from build123d import *

# Parameters (mm, degrees)
F0_W     = 584.2
F0_H     = 136.525
F1_DEPTH = 88.9
F2_R     = 3.81
F3_T     = -2.54


# Not quite as in the source:
# - a shell that OpenCascade refuses in one call is made with other operations: the cavity is built on its own and cut out


with BuildPart() as f1:
    # F0 (on Front) → F1 (new body)
    with BuildSketch(Plane.XZ):
        Rectangle(F0_W, F0_H)
    extrude(amount=F1_DEPTH)

    # F2
    f2_edges = [f1.edges().sort_by_distance(p)[0] for p in [
        (-292.1, -44.45, 68.2625),
        (0, 0, 68.2625),
        (0, -88.9, 68.2625),
        (-292.1, -88.9, 0),
        (0, -88.9, -68.2625),
        (292.1, -88.9, 0),
        (292.1, -44.45, 68.2625),
        (-292.1, 0, 0),
        (-292.1, -44.45, -68.2625),
        (0, 0, -68.2625),
        (292.1, 0, 0),
        (292.1, -44.45, -68.2625),
    ]]
    fillet(f2_edges, radius=F2_R)

    # F3: a shell. OpenCascade refuses it in one call, so the cavity is built on its own and cut out:
    # the body offset inwards by the wall thickness, plus a prism from it out through each open face.
    f3_core = offset(f1.part, amount=F3_T, mode=Mode.PRIVATE)
    f3_exits = [f3_core.faces().sort_by_distance(p)[0] for p in [
        (0, -44.45, 65.7225),
    ]]
    add(f3_core, mode=Mode.SUBTRACT)
    extrude(f3_exits, amount=-F3_T, mode=Mode.SUBTRACT)


solid = f1.part
Read the model definition and answer for the solid it produces. Units are mm, in the model's axes. A direction names the side the tool comes from. Coordinates: 2 decimals unless noted, no trailing zeros. Order: outer loops, then holes, each group sorted by start corner. A loop starts at its lowest first (then second) coordinate and runs counter-clockwise, first axis right, second up. Notation, with made-up numbers: M -39,12.25 L 11,12.25 A20 ccw 11,49.25 Z; hole C 70,-3 d5. An arc over 180 degrees is marked long. Put each result on its own line as item: value. Start each with the question number.
Item 1: Consider probe 1 along Y at (x, z) = (-238, -5.5); probe 2 along X at (y, z) = (-60, 47.5); probe 3 along Z at (x, y) = (226, -82). Determine where each line is inside the solid, lowest interval first. Write a range as [from, to].
Item 2: For faces 4 (the face through (-4, -44, -65.722)), 5 (the face through (-289.56, -44, -1)), 6 (the face through (-4, -44, -68.262)), determine the directions among +Z, -Z, +X, -X, +Y, -Y from which every point of the face is accessible in a straight line to the end or side of a thin tool.
Item 3: Section A-A, the plane z = 39.5 is taken. Determine the outline of the cut face in (x, y).
Item 4: Section C-C, the plane y = -40 is taken. Determine the outline of the cut face in (x, z), plus the area to 3 significant figures.
Item 5: The mould has two halves that part along Y. Classify faces 1 (the face through (-4, -2.54, 1)), 2 (the face through (292.1, -44, -1)), 3 (the face through (-4, -88.9, 1)): +Y half, -Y half, draft (parallel to the pull), parting line (faces both ways), or undercut.
Item 6: Section B-B, the plane x = -232.5 is taken. Determine the outline of the cut face in (y, z), plus the area to 3 significant figures.
Item 7: Given pin 1 Ø6 at (x, y) = (231, -58.5) entering from +Z; pin 2 Ø0.8 at (y, z) = (-35.5, 67.5) entering from -X; pin 3 Ø0.8 at (x, z) = (-63, 67.5) entering from -Y, each flat-ended and moving along its own axis, determine where each tip first touches the part or whether it passes through.
Computed:
1. probe 1: y = [-88.9, -86.36], [-2.54, 0]
1. probe 2: x = [-292.1, -289.56], [289.56, 292.1]
1. probe 3: z = [-68.26, -65.72]
2. face 4: +Z
2. face 5: none
2. face 6: -Z, +X, -X, +Y, -Y
3. outline: M -292.1,-85.09 A3.81 ccw -288.29,-88.9 L 288.29,-88.9 A3.81 ccw 292.1,-85.09 L 292.1,-3.81 A3.81 ccw 288.29,0 L -288.29,0 A3.81 ccw -292.1,-3.81 Z; hole M -289.56,-85.09 A1.27 ccw -288.29,-86.36 L 288.29,-86.36 A1.27 ccw 289.56,-85.09 L 289.56,-3.81 A1.27 ccw 288.29,-2.54 L -288.29,-2.54 A1.27 ccw -289.56,-3.81 Z
4. outline: M -292.1,-64.45 A3.81 ccw -288.29,-68.26 L 288.29,-68.26 A3.81 ccw 292.1,-64.45 L 292.1,64.45 A3.81 ccw 288.29,68.26 L 288.29,65.72 A1.27 cw 289.56,64.45 L 289.56,-64.45 A1.27 cw 288.29,-65.72 L -288.29,-65.72 A1.27 cw -289.56,-64.45 L -289.56,64.45 A1.27 cw -288.29,65.72 L -288.29,68.26 A3.81 ccw -292.1,64.45 Z
4. area: 2,160 mm2
5. face 1: undercut
5. face 2: draft
5. face 3: -Y half
6. outline: M -88.9,-64.45 A3.81 ccw -85.09,-68.26 L -3.81,-68.26 A3.81 ccw 0,-64.45 L 0,64.45 A3.81 ccw -3.81,68.26 L -3.81,65.72 A1.27 cw -2.54,64.45 L -2.54,-64.45 A1.27 cw -3.81,-65.72 L -85.09,-65.72 A1.27 cw -86.36,-64.45 L -86.36,64.45 A1.27 cw -85.09,65.72 L -85.09,68.26 A3.81 ccw -88.9,64.45 Z
6. area: 902 mm2
7. pin 1: stops at z = -65.72
7. pin 2: stops at x = -291.03
7. pin 3: stops at y = -87.83
